from build123d import *

# Parameters (mm, degrees)
F0_W     = 85
F0_H     = 85
F0_R     = 1.8
F2_DEPTH = 5
F1_R     = 1.75
F3_DEPTH = 10


with BuildPart() as f2:
    # F0 (on Top) → F2 (new body)
    with BuildSketch(Plane.XY):
        Rectangle(F0_W, F0_H)
        with Locations((-31.1, -31.1)):
            Circle(F0_R, mode=Mode.SUBTRACT)
        with Locations((31.1, -31.1)):
            Circle(F0_R, mode=Mode.SUBTRACT)
        with Locations((-31.1, 31.1)):
            Circle(F0_R, mode=Mode.SUBTRACT)
        with Locations((31.1, 31.1)):
            Circle(F0_R, mode=Mode.SUBTRACT)
    extrude(amount=F2_DEPTH)

    # F1 (on face) → F3 (cut)
    with BuildSketch(Plane.XY):
        with Locations((-4.47245, 35.938702)):
            Circle(F1_R)
        with Locations((35.938702, -4.47245)):
            Circle(F1_R)
        with Locations((4.47245, -35.938702)):
            Circle(F1_R)
        with Locations((-35.938702, 4.47245)):
            Circle(F1_R)
    extrude(amount=F3_DEPTH, mode=Mode.SUBTRACT)


solid = f2.part
Could you check a few things on this model? Use its own coordinates, in mm. Coordinates: 2 decimals unless noted, no trailing zeros. Order: outer loops, then holes, each group sorted by start corner. A loop starts at its lowest first (then second) coordinate and runs counter-clockwise, first axis right, second up. Notation, with made-up numbers: (-10.5, 47.5) -> (27.5, 47.5) arc R32 cw to (27.5, 73.5) -> close; hole circle Ø8 at (37.25, -21.75). An arc over 180 degrees is marked (long way). One line per item, written item: value. Start each with the question number.
1) Imagine slicing it at A-A on x = -31.1. List the corners of the cut face in (y, z) for me, plus the area to 3 significant figures.
2) If I drill on L1, parallel to Y at x = -31.1, z = 2.75; L2, parallel to X at y = -30, z = 2.35; L3, parallel to Y at x = 32.5, z = 1.35, over which ranges is the centre line in solid material (lowest first)? Write a range as [from, to].
3) I'm going to push a flat-ended pin straight in: pin 1 (3 mm diameter, centred on x = -31.1, y = -31.1, fed in from -Z). Where does the tip first touch, or does it pass through?
4) We'd pull the mould along Y, two halves only. Please class faces 1 (the flat face through (-1, 42.5, 2)), 2 (the cylindrical face through (-30.132, 32.618, 2.465)), 3 (the flat face through (-1, 1, 0)): +Y half, -Y half, draft (parallel to the pull), parting line (faces both ways), or undercut.
Answer list:
1. outline: (-42.5, 0) -> (-32.9, 0) -> (-32.9, 5) -> (-42.5, 5) -> close; (-29.3, 0) -> (29.3, 0) -> (29.3, 5) -> (-29.3, 5) -> close; (32.9, 0) -> (42.5, 0) -> (42.5, 5) -> (32.9, 5) -> close
1. area: 389 mm2
2. L1: y = [-42.5, -32.9], [-29.3, 29.3], [32.9, 42.5]
2. L2: x = [-42.5, -32.52], [-29.68, 29.68], [32.52, 42.5]
2. L3: y = [-42.5, -32.23], [-29.97, 29.97], [32.23, 42.5]
3. pin 1: passes through
4. face 1: +Y half
4. face 2: undercut
4. face 3: draft
